The model under review builds one solid part; all positions refer to its coordinate system, in mm. A direction names the side the tool comes from. Round coordinates to 2 decimals unless told otherwise and drop trailing zeros. Order: outer loops, then holes, each group sorted by start corner. A loop starts at its lowest first (then second) coordinate and runs counter-clockwise, first axis right, second up.
1) Consider section C-C (z = 10.5). Give the boundary of the cut face in (x, y).
2) Machinability: for faces 4 (the face through (-0.921, 4.149, 2.406)), 5 (the face through (0, 3, 7)), 6 (the face through (-6, 0, 11)), which of the approach directions +Z, -Z, +X, -X, +Y, -Y give a long, thin tool a straight path to every point of the face, cutting with its end or side? Answer none if there is none.
3) Consider section A-A (y = 0). Give the boundary of the cut face in (x, z), then the cut area to 3 significant figures.
4) Consider section D-D (z = 1.5). Give the boundary of the cut face in (x, y).
5) To check wall thickness, follow L1, parallel to Y at x = 0, z = 10; L2, parallel to Z at x = 7, y = -0.5. State the ranges of each line that lie inside material, in increasing order.
6) Clearance check with flat-ended pins moving along their axes: P1, Ø2, axis at y = -4, z = 4.5, coming from the +X side; P2, Ø1.5, axis at y = -6, z = 11, coming from the -X side; P3, Ø2, axis at x = -1, z = 11, coming from the +Y side. State where each tip first meets the part, or that it passes through.
7) Mouldability with a two-part tool opening along Z and no side actions: class faces 1 (the face through (-0.867, 3.905, 3.979)), 2 (the face through (-3, -1, 14)), 3 (the face through (-1.73, 7.81, 0.49)) as pulls with the +Z half, pulls with the -Z half, needs draft (parallel to the pull), parting line crosses it, or undercut.
Solid Edge part; units mm, degrees
sketch "Sketch1" plane through (0, 0, 0) normal (0, 0, 1) x (1, 0, 0)
  circle A0 centre (0, 0) radius 8
extrude "Protrusion1" add sketch "Sketch1" along normal blind 14
sketch "Sketch2" plane through (0, 0, 0) normal (0, -1, 0) x (1, 0, 0)
  line L0 (8, 14.2715) -> (6, 14.2715)
  line L1 (6, 14.2715) -> (6, 8)
  line L2 (6, 8) -> (8, 8)
  line L3 (8, 8) -> (8, 14.2715)
  line L4 (4, 5.5) -> (4, 2.5)
  line L5 (4, 2.5) -> (8, 1)
  line L6 (8, 7) -> (8, 1)
  line L7 (4, 5.5) -> (8, 7)
  dimension "D1" = 4
revolve "RevolvedCutout1" cut sketch "Sketch2" angle 360 about axis through (0, 0, 0) along (0, 0, 1)
hole "Hole_1" at (0, 0, 14) direction (0, 0, -1) diameter 6 end through all
Answer below:
1. outline: circle Ø12 at (0, 0); hole circle Ø6 at (0, 0)
2. face 4: none
2. face 5: +Z, -Z
2. face 6: +Z
3. outline: (-8, 0) - (-3, 0) - (-3, 14) - (-6, 14) - (-6, 8) - (-8, 8) - (-8, 7) - (-4, 5.5) - (-4, 2.5) - (-8, 1) - close; (3, 0) - (8, 0) - (8, 1) - (4, 2.5) - (4, 5.5) - (8, 7) - (8, 8) - (6, 8) - (6, 14) - (3, 14) - close
3. area: 80.0 mm2
4. outline: circle Ø13.33 at (0, 0); hole circle Ø6 at (0, 0)
5. L1: y = -6 to -3, 3 to 6
5. L2: z = 0 to 1.37, 6.63 to 8
6. P1: stops at x = 2.65
6. P2: stops at x = -2.9
6. P3: stops at y = 6
7. face 1: undercut
7. face 2: pulls with the +Z half
7. face 3: needs draft
